from build123d import *

# Parameters (mm, degrees)
F0_R     = 5
F1_DEPTH = 3
F0_R_2   = 1.15
F2_DEPTH = 6
F3_DEPTH = 2


with BuildPart() as f1:
    # F0 (on Top) → F1 (new body)
    with BuildSketch(Plane.XY):
        with BuildLine():
            ThreePointArc((6.914658, -3.5), (7.538272, -1.799152), (7.75, 0))
            ThreePointArc((7.75, 0), (7.538272, 1.799152), (6.914658, 3.5))
            ThreePointArc((6.914658, 3.5), (0, 7.75), (-6.914658, 3.5))
            ThreePointArc((-6.914658, 3.5), (-7.75, 0), (-6.914658, -3.5))
            ThreePointArc((-6.914658, -3.5), (0, -7.75), (6.914658, -3.5))
        make_face()
        Circle(F0_R, mode=Mode.SUBTRACT)
        with BuildLine():
            ThreePointArc((-6.914658, -3.5), (-7.75, 0), (-6.914658, 3.5))
            Line((-6.914658, 3.5), (-12.5, 3.5))
            Line((-12.5, 3.5), (-12.5, -3.5))
            Line((-12.5, -3.5), (-6.914658, -3.5))
        make_face()
        with BuildLine():
            ThreePointArc((6.914658, 3.5), (7.538272, 1.799152), (7.75, 0))
            ThreePointArc((7.75, 0), (7.538272, -1.799152), (6.914658, -3.5))
            Line((6.914658, -3.5), (12.5, -3.5))
            Line((12.5, -3.5), (12.5, 3.5))
            Line((12.5, 3.5), (6.914658, 3.5))
        make_face()
    extrude(amount=F1_DEPTH)

    # F0 (on Top) → F2 (join)
    with BuildSketch(Plane.XY):
        with BuildLine():
            ThreePointArc((-6.914658, 3.5), (0, 7.75), (6.914658, 3.5))
            Line((6.914658, 3.5), (12.5, 3.5))
            Line((12.5, 3.5), (12.5, 12.5))
            Line((12.5, 12.5), (-12.5, 12.5))
            Line((-12.5, 12.5), (-12.5, 3.5))
            Line((-12.5, 3.5), (-6.914658, 3.5))
        make_face()
        with Locations((-10.5, 10.5)):
            Circle(F0_R_2, mode=Mode.SUBTRACT)
        with Locations((10.5, 10.5)):
            Circle(F0_R_2, mode=Mode.SUBTRACT)
        with BuildLine():
            Line((12.5, -3.5), (6.914658, -3.5))
            ThreePointArc((6.914658, -3.5), (0, -7.75), (-6.914658, -3.5))
            Line((-6.914658, -3.5), (-12.5, -3.5))
            Line((-12.5, -3.5), (-12.5, -12.5))
            Line((-12.5, -12.5), (12.5, -12.5))
            Line((12.5, -12.5), (12.5, -3.5))
        make_face()
        with Locations((-10.5, -10.5)):
            Circle(F0_R_2, mode=Mode.SUBTRACT)
        with Locations((10.5, -10.5)):
            Circle(F0_R_2, mode=Mode.SUBTRACT)
    extrude(amount=F2_DEPTH)

    # F0 (on Top) → F3 (join)
    with BuildSketch(Plane.XY):
        Circle(F0_R)
    extrude(amount=F3_DEPTH)


solid = f1.part
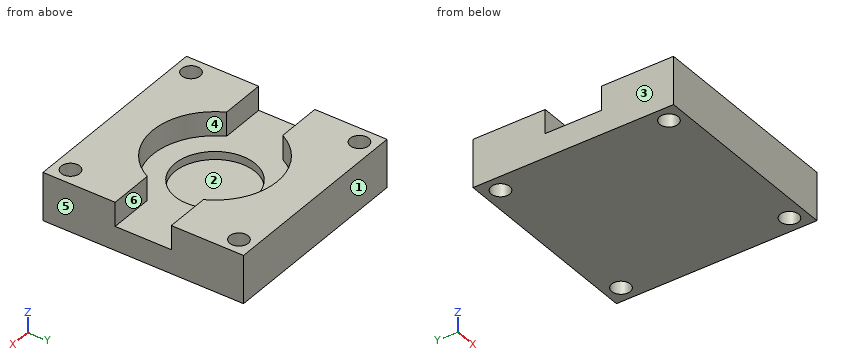
CAD build for the part. Positions are in the model's coordinates, mm. Face numbers are marked on the shaded views. A direction names the side the tool comes from. Give positions to 0.01 mm unless a question says otherwise; leave off trailing zeros. Order: outer loops, then holes, each group sorted by start corner. A loop starts at its lowest first (then second) coordinate and runs counter-clockwise, first axis right, second up. Notation, with made-up numbers: (14, 58.25) -> (61, 58.25) arc R29 ccw to (61, 97.25) -> close; hole circle Ø1 at (76.25, 0). An arc over 180 degrees is marked (long way). Return JSON: item names as keys, results as strings.
Q1. Saw through at D-D (y = 0). Write the cut outline in (x, z), then the cut area to 3 significant figures.
Working result:
{"outline": "(-12.5, 0) -> (12.5, 0) -> (12.5, 3) -> (5, 3) -> (5, 2) -> (-5, 2) -> (-5, 3) -> (-12.5, 3) -> close", "area": "65.0 mm²"}
Q2. Drill centre lines: line 1 (Y direction, x = -10.5, z = 1.7); line 2 (Y direction, x = 9, z = 4.7); line 3 (X direction, y = 11.5, z = 5.2). Where is each one in solid material? Low to high.
Working result:
{"line 1": "-12.5 to -11.65, -9.35 to 9.35, 11.65 to 12.5", "line 2": "-12.5 to -3.5, 3.5 to 12.5", "line 3": "-12.5 to -11.07, -9.93 to 9.93, 11.07 to 12.5"}
Q3. Which spindle directions (+Z, -Z, +X, -X, +Y, -Y) get a long thin tool onto all of the face, cutting with end or side? Do the marked faces 4, 5 and 6. Say none if no direction does.
Working result:
{"face 4": "+Z", "face 5": "+Z, -Z, +X, +Y, -Y", "face 6": "+Z, +X, -X"}
Q4. Saw through at B-B (y = -10.5). Write the cut outline in (x, z), then the cut area to 3 significant figures.
Working result:
{"outline": "(-12.5, 0) -> (-11.65, 0) -> (-11.65, 6) -> (-12.5, 6) -> close; (-9.35, 0) -> (9.35, 0) -> (9.35, 6) -> (-9.35, 6) -> close; (11.65, 0) -> (12.5, 0) -> (12.5, 6) -> (11.65, 6) -> close", "area": "122 mm²"}
Q5. Saw through at A-A (x = 10.5). Write the cut outline in (y, z).
Working result:
{"outline": "(-12.5, 0) -> (-11.65, 0) -> (-11.65, 6) -> (-12.5, 6) -> close; (-9.35, 0) -> (9.35, 0) -> (9.35, 6) -> (3.5, 6) -> (3.5, 3) -> (-3.5, 3) -> (-3.5, 6) -> (-9.35, 6) -> close; (11.65, 0) -> (12.5, 0) -> (12.5, 6) -> (11.65, 6) -> close"}
Q6. Mould opens along Y. For the marked faces 1, 2 and 3 say: pulls with the +Y half, pulls with the -Y half, needs draft (parallel to the pull), parting line crosses it, or undercut.
Working result:
{"face 1": "pulls with the +Y half", "face 2": "undercut", "face 3": "needs draft"}
Q7. Flat gauge pins, fed straight in: pin 1 (1.4 mm diameter, centred on x = 10.5, y = -10.5, fed in from -Z); pin 2 (3 mm diameter, centred on x = 0, y = -2, fed in from +Z); pin 3 (13 mm diameter, centred on x = 0, y = 0, fed in from +Z). Where does each tip first touch, or does it go through?
Working result:
{"pin 1": "through", "pin 2": "z = 2", "pin 3": "z = 3"}
Q8. Saw through at C-C (z = 2.55). Write the cut outline in (x, y).
Working result:
{"outline": "(-12.5, -12.5) -> (12.5, -12.5) -> (12.5, 12.5) -> (-12.5, 12.5) -> close; hole circle Ø2.3 at (-10.5, -10.5); hole circle Ø2.3 at (-10.5, 10.5); hole circle Ø10 at (0, 0); hole circle Ø2.3 at (10.5, -10.5); hole circle Ø2.3 at (10.5, 10.5)"}
